Can you work these out from the model? Positions are in its coordinate system, mm. Face numbers are marked on the shaded views. A direction names the side the tool comes from. Coordinates: 2 decimals unless noted, no trailing zeros. Loops run counter-clockwise (first coordinate to the right, second up) from the corner with the lowest first, then second, coordinate; pieces in that order, holes last.
```python
from build123d import *

# Parameters (mm, degrees)
SKETCH_1_R      = 2.7
EXTRUDE_1_DEPTH = 0.6
SKETCH_5_R      = 0.225
EXTRUDE_2_DEPTH = 10


with BuildPart() as part:
    # Эскиз1 → Бобышка-Вытянуть1 (new body)
    with BuildSketch(Plane(origin=(0, 0, 0), x_dir=(1, 0, 0), z_dir=(0, 1, 0))):
        with Locations(Location((0, 0, 0), (0, 0, 270))):
            Circle(SKETCH_1_R)
    extrude(amount=EXTRUDE_1_DEPTH)

    # Sketch 1 2 → Повернуть1 (revolve)
    with BuildSketch(Plane(origin=(0, 0.6, 0), x_dir=(-0.5248887029964605, 0.85117086972399, 0), z_dir=(0, 0, 1)), mode=Mode.PRIVATE) as revolve_1_sk:
        with BuildLine():
            Line((0, 0), (1.233488452, 2.000251544))
            Line((1.233488452, 2.000251544), (3.361415626, 0.688029786))
            ThreePointArc((3.361415626, 0.688029786), (3.585481802, 0.377802518), (3.52455671, 0))
            Line((3.52455671, 0), (2.553512609, -1.574666109))
            Line((2.553512609, -1.574666109), (0, 0))
        make_face()
    revolve(revolve_1_sk.sketch.rotate(Axis((0, 7.936864243, 0), (0, -1, 0)), 270), axis=Axis((0, 7.936864243, 0), (0, -1, 0)))

    # Эскиз5 → Бобышка-Вытянуть2 (add)
    with BuildSketch(Plane.XZ):
        with Locations(Location((1.27, 0, 0), (0, 0, 90))):
            Circle(SKETCH_5_R)
        with Locations(Location((0, 1.27, 0), (0, 0, 90))):
            Circle(SKETCH_5_R)
        with Locations(Location((0, -1.27, 0), (0, 0, 90))):
            Circle(SKETCH_5_R)
    extrude(amount=EXTRUDE_2_DEPTH)


solid = part.part
```
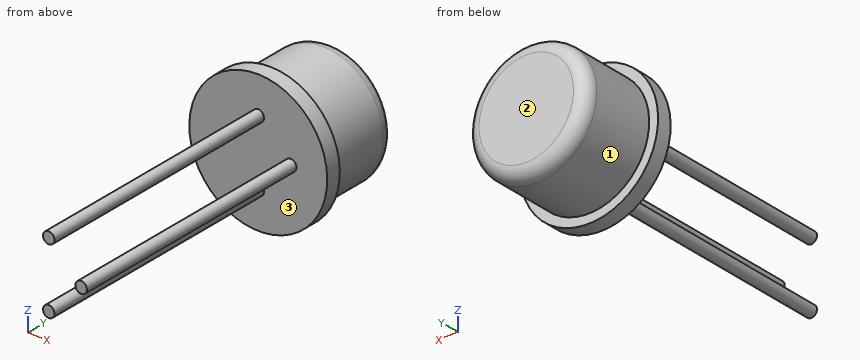
(1) Which directions (+Z, -Z, +X, -X, +Y, -Y) give clear straight access to the entire face, cutting with the end or side of a thin tool? Please do the marked faces 1, 2 and 3.
Check values:
face 1: +Y
face 2: +Z, -Z, +X, -X, +Y
face 3: -Y
(2) I want a section at A-A on x = 0. Write out the boundary of the cut face in (y, z) (3 decimals), then the cut area to 3 significant figures.
Check values:
outline: (-10, -1.495) - (0, -1.495) - (0, -2.7) - (0.6, -2.7) - (0.6, -2.35) - (3.1, -2.35) arc R0.5 ccw to (3.6, -1.85) - (3.6, 1.85) arc R0.5 ccw to (3.1, 2.35) - (0.6, 2.35) - (0.6, 2.7) - (0, 2.7) - (0, 1.495) - (-10, 1.495) - (-10, 1.045) - (0, 1.045) - (0, -1.045) - (-10, -1.045) - close
area: 26.2 mm2
(3) If I drill on probe 1 along Y at (x, z) = (-0.5, -0.25); probe 2 along Z at (x, y) = (0.15, -3.5); probe 3 along Y at (x, z) = (-1.55, 1.85), over which ranges is the centre line in solid material (lowest first)?
Check values:
probe 1: y = 0 to 3.6
probe 2: z = -1.44 to -1.1, 1.1 to 1.44
probe 3: y = 0 to 0.6
(4) I want a section at C-C on z = 0. Write out the boundary of the cut face in (x, y) (3 decimals), then the cut area to 3 significant figures.
Check values:
outline: (-2.7, 0) - (1.045, 0) - (1.045, -10) - (1.495, -10) - (1.495, 0) - (2.7, 0) - (2.7, 0.6) - (2.35, 0.6) - (2.35, 3.1) arc R0.5 ccw to (1.85, 3.6) - (-1.85, 3.6) arc R0.5 ccw to (-2.35, 3.1) - (-2.35, 0.6) - (-2.7, 0.6) - close
area: 21.7 mm2
(5) I'm going to push flat-ended pins straight in: pin 1 (1 mm diameter, centred on x = -0.5, y = -4.5, fed in from +Z) (3 decimals); pin 2 (1 mm diameter, centred on x = 0, z = 1, fed in from -Y); pin 3 (1 mm diameter, centred on y = -6, z = 0.5, fed in from +X) (3 decimals); pin 4 (1 mm diameter, centred on y = -8, z = 1.5, fed in from +X) (3 decimals). Where does each tip first touch, or does it pass through?
Check values:
pin 1: stops at z = 1.495
pin 2: stops at y = -10
pin 3: stops at x = 1.495
pin 4: stops at x = 0.225
(6) I want a section at B-B on y = -0.5. Write out the boundary of the cut face in (x, z) (3 decimals), then the cut area to 3 significant figures.
Check values:
outline: circle Ø0.45 at (0, -1.27); circle Ø0.45 at (0, 1.27); circle Ø0.45 at (1.27, 0)
area: 0.477 mm2
